from build123d import *

# Parameters (mm, degrees)
F0_W      = 81.28
F0_H      = 50.8
F1_DEPTH  = 4
F2_W      = 3
F2_H      = 47.8
F2_H_2    = 3
F2_W_2    = 75.28
F3_DEPTH  = 50.8
F4_W      = 75.28
F4_H      = 47.8
F5_DEPTH  = 4
F6_W      = 3.6
F6_H      = 5
F7_DEPTH  = 5.6
F9_W      = 3.3
F9_H      = 4.5
F10_DEPTH = 9
F11_DEPTH = 3.5


with BuildPart() as f1:
    # F0 (on Front) → F1 (new body)
    with BuildSketch(Plane.XZ):
        Rectangle(F0_W, F0_H)
    extrude(amount=F1_DEPTH)

    # F2 (on face) → F3 (join)
    with BuildSketch(Plane.XZ.offset(4)):
        with Locations((-39.14, 1.5)):
            Rectangle(F2_W, F2_H)
        with Locations((-39.14, -23.9)):
            Rectangle(F2_W, F2_H_2)
        with Locations((0, -23.9)):
            Rectangle(F2_W_2, F2_H_2)
        with Locations((39.14, -23.9)):
            Rectangle(F2_W, F2_H_2)
        with Locations((39.14, 1.5)):
            Rectangle(F2_W, F2_H)
    extrude(amount=F3_DEPTH)

    # F4 (on face) → F5 (join)
    with BuildSketch(Plane.XZ.offset(54.8)):
        Polygon((-40.64, 25.4), (-40.64, -25.4), (40.64, -25.4), (40.64, 25.4), (37.64, 25.4), (37.64, -22.4), (-37.64, -22.4), (-37.64, 25.4), align=None)
        with Locations((0, 1.5)):
            Rectangle(F4_W, F4_H)
    extrude(amount=F5_DEPTH)

    # F6 (on face) → F7 (join)
    with BuildSketch(Plane(origin=(0, 0, 0), x_dir=(-1, 0, 0), z_dir=(0, 1, 0))):
        with Locations((-38.84, 22.9)):
            Rectangle(F6_W, F6_H)
        with Locations((38.84, 22.9)):
            Rectangle(F6_W, F6_H)
    extrude(amount=F7_DEPTH)

    # F9 (on face) → F10 (join)
    with BuildSketch(Plane(origin=(0, 0, 0), x_dir=(-1, 0, 0), z_dir=(0, 1, 0))):
        with Locations((38.99, -1.85)):
            Rectangle(F9_W, F9_H)
        with Locations((-38.99, -1.85)):
            Rectangle(F9_W, F9_H)
    extrude(amount=F10_DEPTH)

    # F8 (on face) → F11 (join)
    with BuildSketch(Plane(origin=(-40.64, 0, 0), x_dir=(0, -1, 0), z_dir=(-1, 0, 0))):
        with BuildLine():
            Line((-8.6013965008, 30.4046550027), (-8.6013965008, 25.4046550027))
            ThreePointArc((-8.6013965008, 25.4046550027), (-7.6846062869, 22.5521456134), (-5.6, 20.4))
            Line((-5.6, 20.4), (-5.6, 25.4))
            ThreePointArc((-5.6, 25.4), (-6.8110562613, 27.7642200981), (-7.1013965008, 30.4046550027))
            Line((-7.1013965008, 30.4046550027), (-8.6013965008, 30.4046550027))
        make_face()
    extrude(amount=-F11_DEPTH)

    # F12: F1 across plane


with BuildPart() as f1_1:
    add(f1.part)
    add(f1.part.mirror(Plane.YZ))


solid = f1_1.part
Could you check a few things on this model? Use its own coordinates, in mm. A direction names the side the tool comes from. Give positions to 0.01 mm unless a question says otherwise; leave off trailing zeros. Order: outer loops, then holes, each group sorted by start corner. A loop starts at its lowest first (then second) coordinate and runs counter-clockwise, first axis right, second up.
Item 1: I need wall thicknesses on line 1 (X direction, y = -7, z = -12.5); line 2 (Y direction, x = 36, z = 24); line 3 (Z direction, x = 9, y = -21.5). Which ranges of each line are inside material? Lowest first, please.
Item 2: If we section it at B-B, the plane y = 3.5: Write out the boundary of the cut face in (x, z).
Item 3: If we section it at C-C, the plane x = -31.5: Write out the boundary of the cut face in (y, z), plus the area to 3 significant figures.
Item 4: If we section it at D-D, the plane y = -10: Write out the boundary of the cut face in (x, z), plus the area to 3 significant figures.
Item 5: If we section it at A-A, the plane z = -6.5: Write out the boundary of the cut face in (x, y).
Item 6: If we mould it in two halves opening along X, with no side actions, what happens to faces 1 (the face through (37.64, -29, 1)), 2 (the face through (40.64, -24, 3)), 3 (the face through (-1, -54.8, 2)), 4 (the face through (-1, -58.8, 0))? For each: pulls with the +X half, pulls with the -X half, needs draft (parallel to the pull), parting line crosses it, or undercut.
Item 7: For faces 5 (the face through (37.34, 4, -2)), 6 (the face through (39, 4, 0.4)), 7 (the face through (-1, -4, 2)), which set-ups out of +Z, -Z, +X, -X, +Y, -Y let a thin tool reach every point of the face, with its end or its side?
Item 8: I'm going to push flat-ended pins straight in: pin 1 (3.5 mm diameter, centred on x = -38, y = 6, fed in from -Z); pin 2 (1.6 mm diameter, centred on x = -39, y = 4.5, fed in from +Z); pin 3 (4 mm diameter, centred on x = 39, z = 28.5, fed in from +Y). Where does each tip first touch, or does it pass through?
Values:
1. line 1: x = -40.64 to -37.64, 37.64 to 40.64
1. line 2: y = -58.8 to -54.8, -4 to 0
1. line 3: z = -25.4 to -22.4
2. outline: (-40.64, -4.1) - (-37.34, -4.1) - (-37.34, 0.4) - (-40.64, 0.4) - close; (-40.64, 20.4) - (-37.04, 20.4) - (-37.04, 25.4) - (-40.64, 25.4) - close; (37.04, 20.4) - (40.64, 20.4) - (40.64, 25.4) - (37.04, 25.4) - close; (37.34, -4.1) - (40.64, -4.1) - (40.64, 0.4) - (37.34, 0.4) - close
3. outline: (-58.8, -25.4) - (0, -25.4) - (0, 25.4) - (-4, 25.4) - (-4, -22.4) - (-54.8, -22.4) - (-54.8, 25.4) - (-58.8, 25.4) - close
3. area: 559 mm2
4. outline: (-40.64, -25.4) - (40.64, -25.4) - (40.64, 25.4) - (37.64, 25.4) - (37.64, -22.4) - (-37.64, -22.4) - (-37.64, 25.4) - (-40.64, 25.4) - close
4. area: 531 mm2
5. outline: (-40.64, -58.8) - (40.64, -58.8) - (40.64, 0) - (-40.64, 0) - close; hole (-37.64, -54.8) - (37.64, -54.8) - (37.64, -4) - (-37.64, -4) - close
6. face 1: undercut
6. face 2: pulls with the +X half
6. face 3: undercut
6. face 4: needs draft
7. face 5: -Z, +Y
7. face 6: +X, -X, +Y
7. face 7: +Z
8. pin 1: stops at z = -4.1
8. pin 2: stops at z = 25.4
8. pin 3: stops at y = 8.6
